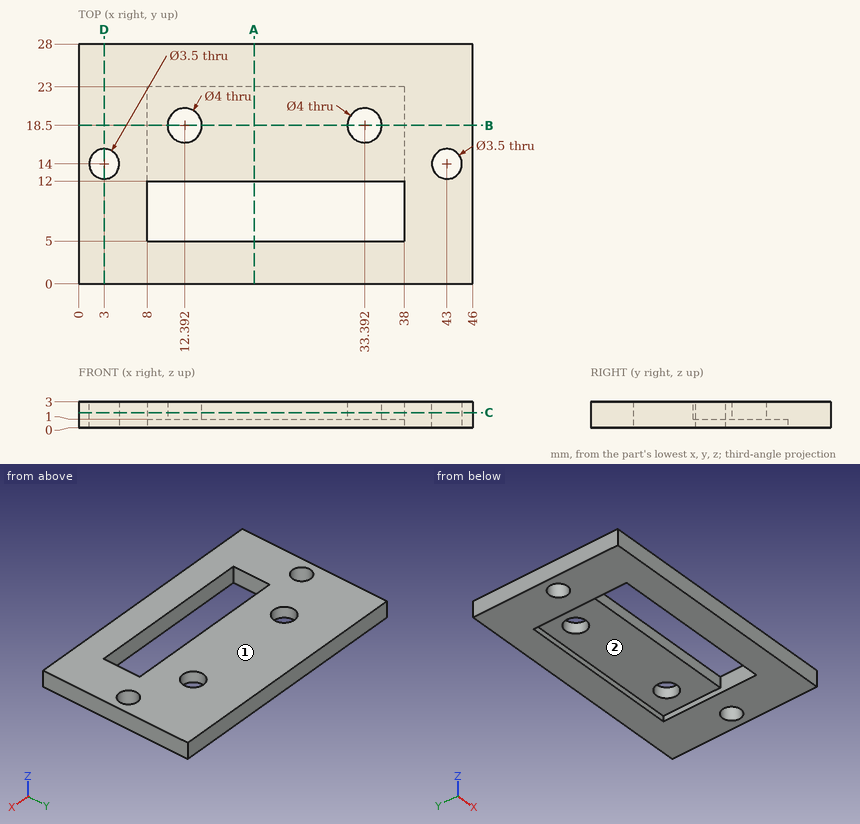
Here's the drawing with two shaded views (mm, measured from the low corner). I have some questions. Give positions to 0.01 mm unless a question says otherwise; leave off trailing zeros. Write each loop counter-clockwise with the first axis right and the second up, starting at its lowest first coordinate (ties: lowest second). Pieces come first, ordered by that corner, then holes. Notation, with made-up numbers: (48, 70) - (88, 70) arc R13 cw to (88, 77) - close; hole circle Ø6 at (23.5, 59). An arc over 180 degrees is marked (long way). Write item = value, one per line. Start each with the question number.
1. Imagine slicing it at C-C (z = 1.75). Please give me the cut outline in (x, y).
2. Please list where these lines run through material, in increasing order: line 1 (Y direction, x = 43, z = 1.25); line 2 (Y direction, x = 23, z = 1.35); line 3 (Y direction, x = 33.5, z = 2.3).
3. Thinking about a two-plate mould opening in X: for the marked faces 1 and 2, which applies, released by +X, released by -X, zero draft, split by the parting line, or undercut?
4. For pin 1 (3 mm diameter, centred on x = 29, y = 13, fed in from -Z); pin 2 (2.5 mm diameter, centred on x = 12.39, y = 18.5, fed in from -Z), each with a flat end and sliding along its axis, tell me the tip position at first contact or that it passes through.
5. Imagine slicing it at D-D (x = 3). Please give me the cut outline in (y, z).
6. Imagine slicing it at A-A (x = 20.5). Please give me the cut outline in (y, z), and give its area (3 significant figures).
7. Imagine slicing it at B-B (y = 18.5). Please give me the cut outline in (x, z).
Worked answers:
q1.outline = (0, 0) - (46, 0) - (46, 28) - (0, 28) - close; hole circle Ø3.5 at (3, 14); hole (8, 5) - (38, 5) - (38, 12) - (8, 12) - close; hole circle Ø4 at (12.39, 18.5); hole circle Ø4 at (33.39, 18.5); hole circle Ø3.5 at (43, 14)
q2.line_1 = 0 to 12.25, 15.75 to 28
q2.line_2 = 0 to 5, 12 to 28
q2.line_3 = 0 to 5, 12 to 16.5, 20.5 to 28
q3.face_1 = zero draft
q3.face_2 = undercut
q4.pin_1 = 1
q4.pin_2 = through
q5.outline = (0, 0) - (12.25, 0) - (12.25, 3) - (0, 3) - close; (15.75, 0) - (28, 0) - (28, 3) - (15.75, 3) - close
q6.outline = (0, 0) - (5, 0) - (5, 3) - (0, 3) - close; (12, 1) - (23, 1) - (23, 0) - (28, 0) - (28, 3) - (12, 3) - close
q6.area = 52.0 mm2
q7.outline = (0, 0) - (8, 0) - (8, 1) - (10.39, 1) - (10.39, 3) - (0, 3) - close; (14.39, 1) - (31.39, 1) - (31.39, 3) - (14.39, 3) - close; (35.39, 1) - (38, 1) - (38, 0) - (46, 0) - (46, 3) - (35.39, 3) - close
